Check sheet for the modelled part. Datum: model origin and axes. Units: mm. A direction names the side the tool comes from. Round coordinates to 2 decimals unless told otherwise and drop trailing zeros. Write each loop counter-clockwise with the first axis right and the second up, starting at its lowest first coordinate (ties: lowest second). Pieces come first, ordered by that corner, then holes. Notation, with made-up numbers: M 41.25,63 L 50.25,63 A27 cw 50.25,100 Z; hole C 63,-4 d9. An arc over 180 degrees is marked long. One line per item, written item: value.
from build123d import *

# Parameters (mm, degrees)
EXTRUDE_1_DEPTH     = 2
SKETCH_2_W          = 2
SKETCH_2_H          = 20
EXTRUDE_2_DEPTH     = 40
FILLET_1_R          = 3
SKETCH_4_W          = 25
SKETCH_4_H          = 1.2
EXTRUDE_3_DEPTH     = 40
FILLET_2_R          = 3
SKETCH_6_R          = 4.5
SKETCH_6_R_2        = 1.5
CUT_EXTRUDE_2_DEPTH = 62.692787261
SKETCH_7_R          = 1
CUT_EXTRUDE_3_DEPTH = 59.857879676


with BuildPart() as part:
    # 草图1 → 凸台-拉伸1 (new body)
    with BuildSketch(Plane(origin=(0, 0, 0), x_dir=(1, 0, 0), z_dir=(0, 1, 0))):
        Polygon((12.5, -10), (12.5, -19), (-12.5, -19), (-12.5, -10), (-20.5, -10), (-20.5, 10), (-12.5, 10), (-12.5, 19), (12.5, 19), (12.5, 10), (20.5, 10), (20.5, -10), align=None)
    extrude(amount=EXTRUDE_1_DEPTH)

    # 草图2 → 凸台-拉伸2 (add)
    with BuildSketch(Plane(origin=(0, 2, 0), x_dir=(1, 0, 0), z_dir=(0, 1, 0))):
        with Locations((-19.5, 0)):
            Rectangle(SKETCH_2_W, SKETCH_2_H)
        with Locations((19.5, 0)):
            Rectangle(SKETCH_2_W, SKETCH_2_H)
    extrude(amount=EXTRUDE_2_DEPTH)

    # 圆角1
    fillet_1_edges = [part.edges().sort_by_distance(p)[0] for p in [
        (-20.5, 0, 0),
        (20.5, 0, 0),
        (-18.5, 2, 0),
        (18.5, 2, 0),
    ]]
    fillet(fillet_1_edges, radius=FILLET_1_R)

    # 草图4 → 凸台-拉伸3 (add)
    with BuildSketch(Plane.XZ):
        with Locations((0, 18.4)):
            Rectangle(SKETCH_4_W, SKETCH_4_H)
        with Locations((0, -18.4)):
            Rectangle(SKETCH_4_W, SKETCH_4_H)
    extrude(amount=EXTRUDE_3_DEPTH)

    # 圆角2
    fillet_2_edges = [part.edges().sort_by_distance(p)[0] for p in [
        (0, 2, -19),
        (0, 2, 19),
        (0, 0, 17.8),
        (0, 0, -17.8),
    ]]
    fillet(fillet_2_edges, radius=FILLET_2_R)

    # 草图6 → 切除-拉伸2 (cut, through all)
    with BuildSketch(Plane.ZY.offset(20.5)):
        with Locations((0, 22)):
            Circle(SKETCH_6_R)
        with Locations((0, 15)):
            Circle(SKETCH_6_R_2)
        with Locations((-7, 22)):
            Circle(SKETCH_6_R_2)
        with Locations((0, 29)):
            Circle(SKETCH_6_R_2)
        with Locations((7, 22)):
            Circle(SKETCH_6_R_2)
        with BuildLine():
            Line((-10, 22), (-10, 42))
            Line((-10, 42), (10, 42))
            Line((10, 42), (10, 22))
            ThreePointArc((10, 22), (0, 32), (-10, 22))
        make_face()
    extrude(amount=-CUT_EXTRUDE_2_DEPTH, mode=Mode.SUBTRACT)

    # 草图7 → 切除-拉伸3 (cut, through all)
    with BuildSketch(Plane.XY.offset(19)):
        with Locations((-10.25, -30.35)):
            Circle(SKETCH_7_R)
        with Locations((-10.25, -9.65)):
            Circle(SKETCH_7_R)
        with Locations((10.25, -9.65)):
            Circle(SKETCH_7_R)
        with Locations((10.25, -30.35)):
            Circle(SKETCH_7_R)
        with BuildLine():
            Line((-12.5, -33), (-9.746794345, -33))
            ThreePointArc((-9.746794345, -33), (0, -28), (9.746794345, -33))
            Line((9.746794345, -33), (12.5, -33))
            Line((12.5, -33), (12.5, -40))
            Line((12.5, -40), (-12.5, -40))
            Line((-12.5, -40), (-12.5, -33))
        make_face()
    extrude(amount=-CUT_EXTRUDE_3_DEPTH, mode=Mode.SUBTRACT)


solid = part.part
Q1. Sectioned sample at C-C on x = 10.5. Enter the section's corners in (y, z), and give its area (3 significant figures).
Completed:
outline: M -33,-19 L -31.32,-19 L -31.32,-17.8 L -33,-17.8 Z; M -33,17.8 L -31.32,17.8 L -31.32,19 L -33,19 Z; M -29.38,-19 L -10.62,-19 L -10.62,-17.8 L -29.38,-17.8 Z; M -29.38,17.8 L -10.62,17.8 L -10.62,19 L -29.38,19 Z; M -8.68,-19 L -1,-19 A3 ccw 2,-16 L 2,16 A3 ccw -1,19 L -8.68,19 L -8.68,17.8 L -3,17.8 A3 cw 0,14.8 L 0,-14.8 A3 cw -3,-17.8 L -8.68,-17.8 Z
area: 146 mm^2
Q2. Scan lines: line 1 (X direction, y = 19, z = -8.5); line 2 (Z direction, x = -3, y = -25); line 3 (Y direction, x = 19.9, z = 0). Record each from-to range of solid material in increasing order. Write a range as [from, to].
Completed:
line 1: [-20.5, -18.5], [18.5, 20.5]
line 2: [-19, -17.8], [17.8, 19]
line 3: [1.2, 13.5], [16.5, 17.5], [26.5, 27.5], [30.5, 32]
Q3. Depth check by flat-ended pin: P1, Ø1.8, axis at x = 10.25, y = -30.35, coming from the -Z side; P2, Ø1.5, axis at x = -6.5, z = -8.5, coming from the -Y side; P3, Ø4, axis at y = 22, z = -7, coming from the -X side; P4, Ø4.5, axis at y = -10.5, z = 16, coming from the -X side. Enter the tip coordinate at first touch or a pass-through.
Completed:
P1: through
P2: y = 0
P3: x = -20.5
P4: x = -12.5
Q4. Sectioned sample at B-B on z = 7. Enter the section's corners in (x, y), and give its area (3 significant figures).
Completed:
outline: M -20.5,3 A3 ccw -17.5,0 L 17.5,0 A3 ccw 20.5,3 L 20.5,20.5 L 18.5,20.5 L 18.5,5 A3 cw 15.5,2 L -15.5,2 A3 cw -18.5,5 L -18.5,20.5 L -20.5,20.5 Z; M -20.5,23.5 L -18.5,23.5 L -18.5,29.14 L -20.5,29.14 Z; M 18.5,23.5 L 20.5,23.5 L 20.5,29.14 L 18.5,29.14 Z
area: 179 mm^2
Q5. Sectioned sample at A-A on y = -4.5. Enter the section's corners in (x, z), and give its area (3 significant figures).
Completed:
outline: M -12.5,-19 L 12.5,-19 L 12.5,-17.8 L -12.5,-17.8 Z; M -12.5,17.8 L 12.5,17.8 L 12.5,19 L -12.5,19 Z
area: 60.0 mm^2
Q6. Sectioned sample at D-D on z = 0. State how many separate pieces and enclosed holes the cut face has, and give its area (3 significant figures).
Completed:
separate pieces: 7
enclosed holes: 0
area: 142 mm^2
Q7. Draft check along Y on faces 5 (the cylindrical face through (19.486, 30.487, -0.195)), 6 (the flat face through (0, -17, 19)), 7 (the cylindrical face through (19.64, 0.9, 0.14)). Enter one of: pulls with the +Y half, pulls with the -Y half, needs draft (parallel to the pull), parting line crosses it, or undercut.
Completed:
face 5: undercut
face 6: needs draft
face 7: pulls with the -Y half
Q8. Access from +Z, -Z, +X, -X, +Y, -Y to the whole of each face (thin tool, end or side, straight path). Record for faces 1 (the flat face through (12.5, -12, 18)), 2 (the flat face through (-18.5, 15, 2)), 3 (the flat face through (0, -18, 17.8)), 4 (the flat face through (19, 9, -10)).
Completed:
face 1: +Z, +X, +Y, -Y
face 2: +Z, -Z, +Y
face 3: +X, -X, -Y
face 4: -Z, +X, +Y, -Y
